from build123d import *

# Parameters (mm, degrees)
SKETCH1_W           = 19.6
SKETCH1_H           = 21.4
SKETCH1_R           = 1.7
BOSS_EXTRUDE1_DEPTH = 4
SKETCH3_W           = 19.6
SKETCH3_H           = 16
BOSS_EXTRUDE2_DEPTH = 4
FILLET1_R           = 1.5


with BuildPart() as part:
    # Sketch1 → Boss-Extrude1 (new body)
    with BuildSketch(Plane.XY):
        with Locations((0, -5.7)):
            Rectangle(SKETCH1_W, SKETCH1_H)
        with Locations((-4.8, 0)):
            Circle(SKETCH1_R, mode=Mode.SUBTRACT)
        with Locations((4.8, 0)):
            Circle(SKETCH1_R, mode=Mode.SUBTRACT)
    extrude(amount=BOSS_EXTRUDE1_DEPTH)

    # Sketch3 → Boss-Extrude2 (add)
    with BuildSketch(Plane.XZ.offset(16.4)):
        with Locations((0, -4)):
            Rectangle(SKETCH3_W, SKETCH3_H)
    extrude(amount=BOSS_EXTRUDE2_DEPTH)

    # Fillet1
    fillet1_edges = [part.edges().sort_by_distance(p)[0] for p in [
        (0, -16.4, 0),
    ]]
    fillet(fillet1_edges, radius=FILLET1_R)


solid = part.part
CAD build for the part. Positions are in the model's coordinates, mm. A direction names the side the tool comes from. Give positions to 0.01 mm unless a question says otherwise; leave off trailing zeros. Loops run counter-clockwise (first coordinate to the right, second up) from the corner with the lowest first, then second, coordinate; pieces in that order, holes last. Notation, with made-up numbers: M 21,41 L 61,41 A23 cw 61,64 Z; hole C -23.5,52 d9. An arc over 180 degrees is marked long. One line per question, with ' | ' between items. Start each with the question number.
1. Probe L1, parallel to Y at x = -4.8, z = 3.15; L2, parallel to Z at x = 8.75, y = -4.25; L3, parallel to Y at x = 1.75, z = -3.25. List the from-to ranges inside material, lowest first. Write a range as from..to.
2. Flat gauge pin, fed straight in: pin 1 (3 mm diameter, centred on x = -3, z = -8.5, fed in from +Y). Where does the tip first touch, or does it go through?
3. Saw through at D-D on y = -13.25. Give the cut face in (x, z).
4. 3-axis set-ups, long thin cutter, end or side, ignore diameter. For faces 5 (the face through (0, -5, 0)), 6 (the face through (0, -18, -12)): which of +Z, -Z, +X, -X, +Y, -Y reach the whole face in a straight line?
5. Saw through at C-C on x = -8.5. Give the cut face in (y, z).
6. Saw through at B-B on y = 0. Give the cut face in (x, z), plus the area to 3 significant figures.
7. Two-plate mould, pull along X, no slides. Class faces 1 (the face through (-3.23, -0.65, 1.97)), 2 (the face through (0.14, -15.97, -0.45)), 3 (the face through (6.37, -0.65, 1.97)), 4 (the face through (9.8, -11, 1)): pulls with the +X half, pulls with the -X half, needs draft (parallel to the pull), parting line crosses it, or undercut.
8. Saw through at A-A on x = -4.8. Give the cut face in (y, z), plus the area to 3 significant figures.
Result sheet:
1) L1: y = -20.4..-1.7, 1.7..5 | L2: z = 0..4 | L3: y = -20.4..-16.4
2) pin 1: stops at y = -16.4
3) outline: M -9.8,0 L 9.8,0 L 9.8,4 L -9.8,4 Z
4) face 5: -Z, +X, -X, +Y | face 6: -Z, +X, -X, +Y, -Y
5) outline: M -20.4,-12 L -16.4,-12 L -16.4,-1.5 A1.5 cw -14.9,0 L 5,0 L 5,4 L -20.4,4 Z
6) outline: M -9.8,0 L -6.5,0 L -6.5,4 L -9.8,4 Z; M -3.1,0 L 3.1,0 L 3.1,4 L -3.1,4 Z; M 6.5,0 L 9.8,0 L 9.8,4 L 6.5,4 Z | area: 51.2 mm^2
7) face 1: undercut | face 2: needs draft | face 3: undercut | face 4: pulls with the +X half
8) outline: M -20.4,-12 L -16.4,-12 L -16.4,-1.5 A1.5 cw -14.9,0 L -1.7,0 L -1.7,4 L -20.4,4 Z; M 1.7,0 L 5,0 L 5,4 L 1.7,4 Z | area: 136 mm^2
